from build123d import *

# Parameters (mm, degrees)
F1_DEPTH = 80
F2_R     = 25.0450733491
F3_DEPTH = 2
F4_SCALE = 1.5


with BuildPart() as f1:
    # F0 (on Top) → F1 (new body)
    with BuildSketch(Plane.XY):
        with BuildLine():
            ThreePointArc((-83.9803607371, -38.2521874792), (-66.8806784634, -30.5992095312), (-59.8739669949, -13.2247109851))
            ThreePointArc((-59.8739669949, -13.2247109851), (-102.2138217774, 4.8900960587), (-86.0784208338, -38.2429350617))
            Line((-86.0784208338, -38.2429350617), (-86.0784208338, -36.0403462646))
            ThreePointArc((-86.0784208338, -36.0403462646), (-100.6577068059, 3.3340255104), (-62.0739669949, -13.2247109851))
            ThreePointArc((-62.0739669949, -13.2247109851), (-68.4366014954, -29.0432629394), (-83.9803607371, -36.0504915177))
            Line((-83.9803607371, -36.0504915177), (-83.9803607371, -38.2521874792))
        make_face()
        with BuildLine():
            Line((-86.0784208338, -36.0403462646), (-86.0784208338, -38.2429350617))
            ThreePointArc((-86.0784208338, -38.2429350617), (-85.0294877149, -38.2695407997), (-83.9803607371, -38.2521874792))
            Line((-83.9803607371, -38.2521874792), (-83.9803607371, -36.0504915177))
            ThreePointArc((-83.9803607371, -36.0504915177), (-85.029507314, -36.0695172521), (-86.0784208338, -36.0403462646))
        make_face()
        with BuildLine():
            Line((-86.0784208338, -12.1068419315), (-86.0784208338, -36.0403462646))
            ThreePointArc((-86.0784208338, -36.0403462646), (-85.029507314, -36.0695172521), (-83.9803607371, -36.0504915177))
            Line((-83.9803607371, -36.0504915177), (-83.9803607371, -12.1068419315))
            Line((-83.9803607371, -12.1068419315), (-74.5387463539, -12.1068419315))
            add(Edge.make_bspline(
                [(-74.5387463539, -9.9696172834), (-73.2151210172, -9.9696172834), (-73.2151210172, -12.1068419315), (-74.5387463539, -12.1068419315)],
                knots=[0, 0, 0, 0, 2.1372246482, 2.1372246482, 2.1372246482, 2.1372246482], degree=3))
            Line((-74.5387463539, -9.9696172834), (-83.9803607371, -9.9696172834))
            add(Edge.make_bspline(
                [(-83.9803607371, -9.9696172834), (-84.0809768118, -3.6797905773), (-89.3996719456, 1.1776616923), (-97.2777081452, 0.2270288754)],
                knots=[0, 0, 0, 0, 16.75682073, 16.75682073, 16.75682073, 16.75682073], degree=3))
            add(Edge.make_bspline(
                [(-98.1584286764, -0.7088489999), (-98.0651277816, -0.131296323), (-97.7239810489, 0.1096969641), (-97.2777081452, 0.2270288754)],
                knots=[0, 0, 0, 0, 1.285121026, 1.285121026, 1.285121026, 1.285121026], degree=3))
            add(Edge.make_bspline(
                [(-86.0784208338, -12.1068419315), (-94.3202596093, -11.7972125657), (-99.1570433309, -6.8904892511), (-98.1584286764, -0.7088489999)],
                knots=[0, 0, 0, 0, 16.6084566517, 16.6084566517, 16.6084566517, 16.6084566517], degree=3))
        make_face()
        with BuildLine():
            add(Edge.make_bspline(
                [(-86.0784208338, -9.9696172834), (-86.3917425183, -3.4782894727), (-91.9644045086, -1.3975845126), (-96.120710429, -1.8510752765)],
                knots=[0, 0, 0, 0, 12.9134931227, 12.9134931227, 12.9134931227, 12.9134931227], degree=3))
            add(Edge.make_bspline(
                [(-96.120710429, -1.8510752765), (-95.9267848545, -7.8749013541), (-90.8607281187, -9.7746726897), (-86.0784208338, -9.9696172834)],
                knots=[0, 0, 0, 0, 12.9134931227, 12.9134931227, 12.9134931227, 12.9134931227], degree=3))
        make_face(mode=Mode.SUBTRACT)
    extrude(amount=F1_DEPTH)

    # F2 (on face) → F3 (join)
    with BuildSketch(Plane(origin=(0, 0, 0), x_dir=(1, 0, 0), z_dir=(0, 0, -1))):
        with Locations((-84.919040344, 13.2247109851)):
            Circle(F2_R)
    extrude(amount=F3_DEPTH)


with BuildPart() as f1_1:
    # F4: moved
    add(f1.part.scale(F4_SCALE).moved(Location((41.9901803686, 6.0534209658, -40))))


solid = f1_1.part
Design review of the part built by this model. Coordinates are the model's own, in mm. A direction names the side the tool comes from. Coordinates: 2 decimals unless noted, no trailing zeros. Write each loop counter-clockwise with the first axis right and the second up, starting at its lowest first coordinate (ties: lowest second). Pieces come first, ordered by that corner, then holes. Notation, with made-up numbers: (8, 31) -> (17, 31) arc R31 ccw to (17, 61) -> close; hole circle Ø2 at (37, -30.5). An arc over 180 degrees is marked (long way). Write each question's results on one line, items separated by ' | '. Start each with the question number.
(1) Tool access review of faces 3 (the face through (-86, -14, 80)), 4 (the face through (-83.98, -30, 19)): name each direction out of +Z, -Z, +X, -X, +Y, -Y from which nothing blocks a thin tool from reaching the whole face with its end or side.
(2) The part is to be moulded in two halves that separate along X. For faces 1 (the face through (-77, -8.901, 19)), 2 (the face through (-86, -14, -43)), say which applies: pulls with the +X half, pulls with the -X half, needs draft (parallel to the pull), parting line crosses it, or undercut.
(3) Take a section at A-A on x = -81. Write out the cut boundary in (y, z), and give its area (3 significant figures).
(4) Take a section at D-D on x = -66.5. Write out the cut boundary in (y, z).
(5) For line 1 along X through (y, z) = (-14.5, 43.5); line 2 along X through (y, z) = (-31.5, 1); line 3 along X through (y, z) = (-2.5, 66.5), list the stretches that pass through material, from the lowest coordinate up. Write a range as from..to.
(6) Clearance check with flat-ended pins moving along their axes: P1, Ø10, axis at x = -63.5, z = -12, coming from the -Y side; P2, Ø12, axis at y = -31.5, z = 30, coming from the +X side; P3, Ø18, axis at y = -26, z = -9, coming from the +X side. State where each tip first meets the part, or that it passes through.
(7) Take a section at B-B on y = -22. Write out the cut boundary in (x, z).
(8) Take a section at C-C on z = 20. Give the number of separate pieces and of enclosed holes in the cut face, and give its area (3 significant figures).
Results found:
1) face 3: +Z, +X, -X, +Y, -Y | face 4: +Z
2) face 1: undercut | face 2: needs draft
3) outline: (-51.09, -43) -> (23.53, -43) -> (23.53, 80) -> (20.2, 80) -> (20.2, -40) -> (-8.9, -40) -> (-8.9, 80) -> (-12.11, 80) -> (-12.11, -40) -> (-47.77, -40) -> (-47.77, 80) -> (-51.09, 80) -> close | area: 1,410 mm2
4) outline: (-46.26, -43) -> (18.69, -43) -> (18.69, 80) -> (14.81, 80) -> (14.81, -40) -> (-42.38, -40) -> (-42.38, 80) -> (-46.26, 80) -> close
5) line 1: x = -122.95..-119.65, -87.13..-83.98, -51.13..-47.83 | line 2: x = -118.52..-114.72, -87.13..-83.98, -56.06..-52.26 | line 3: x = -121.22..-117.74, -104.42..-100.66, -88.98..-85.42, -53.03..-49.56
6) P1: stops at y = -47.34 | P2: stops at x = -49.69 | P3: stops at x = -47.96
7) outline: (-122.05, -43) -> (-48.73, -43) -> (-48.73, 80) -> (-52.12, 80) -> (-52.12, -40) -> (-83.98, -40) -> (-83.98, 80) -> (-87.13, 80) -> (-87.13, -40) -> (-118.66, -40) -> (-118.66, 80) -> (-122.05, 80) -> close
8) separate pieces: 1 | enclosed holes: 2 | area: 1,080 mm2
